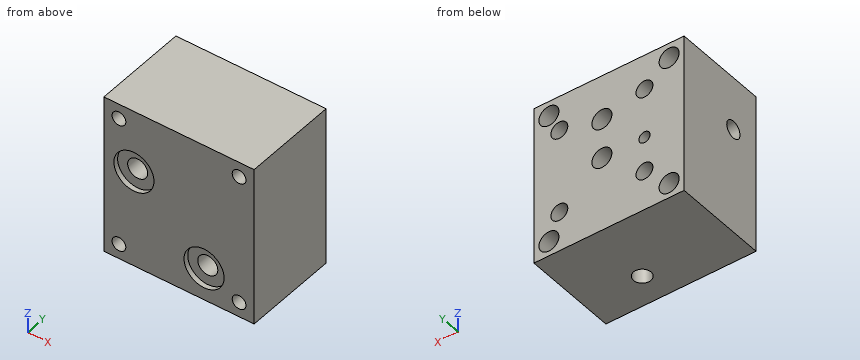
from build123d import *

# Parameters (mm, degrees)
SKETCH1_W           = 95.25
SKETCH1_H           = 101.6
BOSS_EXTRUDE1_DEPTH = 30.1625
CUT_EXTRUDE2_START  = 30.1625
SKETCH2_R           = 4.3688
CUT_EXTRUDE2_DEPTH  = 101.6
CUT_EXTRUDE4_START  = 30.1625
SKETCH3_R           = 6.35
CUT_EXTRUDE4_DEPTH  = 25.4
CUT_EXTRUDE6_START  = 30.1625
SKETCH4_R           = 5.3578125
CUT_EXTRUDE6_DEPTH  = 20.32
CUT_EXTRUDE8_START  = 30.1625
SKETCH5_R           = 6.35
CUT_EXTRUDE8_DEPTH  = 45.72
CUT_EXTRUDE10_START = 30.1625
SKETCH6_R           = 3.556
CUT_EXTRUDE10_DEPTH = 7.9375
CUT_EXTRUDE12_START = -47.625
SKETCH7_R           = 5.55625
CUT_EXTRUDE12_DEPTH = 53.34
CUT_EXTRUDE14_START = -50.8
SKETCH8_R           = 5.55625
CUT_EXTRUDE14_DEPTH = 53.34
CUT_EXTRUDE16_START = -30.1625
SKETCH9_R           = 6.35
CUT_EXTRUDE16_DEPTH = 27.94
CUT_EXTRUDE18_START = -30.1625
SKETCH10_R          = 12.7127
CUT_EXTRUDE18_DEPTH = 3.1242


with BuildPart() as part:
    # Sketch1 → Boss-Extrude1 (new, symmetric)
    with BuildSketch(Plane(origin=(0, 0, 0), x_dir=(1, 0, 0), z_dir=(0, 1, 0))):
        Rectangle(SKETCH1_W, SKETCH1_H)
    extrude(amount=BOSS_EXTRUDE1_DEPTH, both=True)

    # Sketch2 → Cut-Extrude2 (cut)
    with BuildSketch(Plane(origin=(0, 0, 0), x_dir=(1, 0, 0), z_dir=(0, 1, 0)).offset(CUT_EXTRUDE2_START)):
        with Locations(Location((-38.1, -41.275, 0), (0, 0, 270))):
            Circle(SKETCH2_R)
        with Locations(Location((38.1, -41.275, 0), (0, 0, 270))):
            Circle(SKETCH2_R)
        with Locations(Location((-38.1, 41.275, 0), (0, 0, 270))):
            Circle(SKETCH2_R)
        with Locations(Location((38.1, 41.275, 0), (0, 0, 270))):
            Circle(SKETCH2_R)
    extrude(amount=-CUT_EXTRUDE2_DEPTH, mode=Mode.SUBTRACT)

    # Sketch3 → Cut-Extrude4 (cut)
    with BuildSketch(Plane(origin=(0, 0, 0), x_dir=(1, 0, 0), z_dir=(0, 1, 0)).offset(CUT_EXTRUDE4_START)):
        with Locations(Location((-38.1, -41.275, 0), (0, 0, 270))):
            Circle(SKETCH3_R)
        with Locations(Location((38.1, -41.275, 0), (0, 0, 270))):
            Circle(SKETCH3_R)
        with Locations(Location((-38.1, 41.275, 0), (0, 0, 270))):
            Circle(SKETCH3_R)
        with Locations(Location((38.1, 41.275, 0), (0, 0, 270))):
            Circle(SKETCH3_R)
    extrude(amount=-CUT_EXTRUDE4_DEPTH, mode=Mode.SUBTRACT)

    # Sketch4 → Cut-Extrude6 (cut)
    with BuildSketch(Plane(origin=(0, 0, 0), x_dir=(1, 0, 0), z_dir=(0, 1, 0)).offset(CUT_EXTRUDE6_START)):
        with Locations(Location((-22.479, -28.575, 0), (0, 0, 270))):
            Circle(SKETCH4_R)
        with Locations(Location((31.496, -28.575, 0), (0, 0, 270))):
            Circle(SKETCH4_R)
        with Locations(Location((-22.479, 25.4, 0), (0, 0, 270))):
            Circle(SKETCH4_R)
        with Locations(Location((31.496, 25.4, 0), (0, 0, 270))):
            Circle(SKETCH4_R)
    extrude(amount=-CUT_EXTRUDE6_DEPTH, mode=Mode.SUBTRACT)

    # Sketch5 → Cut-Extrude8 (cut)
    with BuildSketch(Plane(origin=(0, 0, 0), x_dir=(1, 0, 0), z_dir=(0, 1, 0)).offset(CUT_EXTRUDE8_START)):
        with Locations(Location((4.5085, -22.225, 0), (0, 0, 270))):
            Circle(SKETCH5_R)
        with Locations(Location((4.5085, 3.175, 0), (0, 0, 270))):
            Circle(SKETCH5_R)
    extrude(amount=-CUT_EXTRUDE8_DEPTH, mode=Mode.SUBTRACT)

    # Sketch6 → Cut-Extrude10 (cut)
    with BuildSketch(Plane(origin=(0, 0, 0), x_dir=(1, 0, 0), z_dir=(0, 1, 0)).offset(CUT_EXTRUDE10_START)):
        with Locations(Location((-22.479, 3.175, 0), (0, 0, 270))):
            Circle(SKETCH6_R)
    extrude(amount=-CUT_EXTRUDE10_DEPTH, mode=Mode.SUBTRACT)

    # Sketch7 → Cut-Extrude12 (cut)
    with BuildSketch(Plane(origin=(0, 0, 0), x_dir=(0, 0, -1), z_dir=(1, 0, 0)).offset(CUT_EXTRUDE12_START)):
        with Locations(Location((-16.637, -11.1125, 0), (0, 0, 233.130102354))):
            Circle(SKETCH7_R)
    extrude(amount=CUT_EXTRUDE12_DEPTH, mode=Mode.SUBTRACT)

    # Sketch8 → Cut-Extrude14 (cut)
    with BuildSketch(Plane.XY.offset(CUT_EXTRUDE14_START)):
        with Locations(Location((10.16, -11.1125, 0), (0, 0, 233.130102354))):
            Circle(SKETCH8_R)
    extrude(amount=CUT_EXTRUDE14_DEPTH, mode=Mode.SUBTRACT)

    # Sketch9 → Cut-Extrude16 (cut)
    with BuildSketch(Plane(origin=(0, 0, 0), x_dir=(1, 0, 0), z_dir=(0, 1, 0)).offset(CUT_EXTRUDE16_START)):
        with Locations(Location((-28.575, -11.1125, 0), (0, 0, 270))):
            Circle(SKETCH9_R)
        with Locations(Location((15.875, 30.1625, 0), (0, 0, 270))):
            Circle(SKETCH9_R)
    extrude(amount=CUT_EXTRUDE16_DEPTH, mode=Mode.SUBTRACT)

    # Sketch10 → Cut-Extrude18 (cut)
    with BuildSketch(Plane(origin=(0, 0, 0), x_dir=(1, 0, 0), z_dir=(0, 1, 0)).offset(CUT_EXTRUDE18_START)):
        with Locations(Location((-28.575, -11.1125, 0), (0, 0, 270))):
            Circle(SKETCH10_R)
        with Locations(Location((15.875, 30.1625, 0), (0, 0, 270))):
            Circle(SKETCH10_R)
    extrude(amount=CUT_EXTRUDE18_DEPTH, mode=Mode.SUBTRACT)


solid = part.part
Work out the finished part from the listing and answer in its coordinate system (mm). Round coordinates to 2 decimals unless told otherwise and drop trailing zeros. Write each loop counter-clockwise with the first axis right and the second up, starting at its lowest first coordinate (ties: lowest second). Pieces come first, ordered by that corner, then holes. Notation, with made-up numbers: (-32, 76.5) - (8, 76.5) arc R31 cw to (8, 105.5) - close; hole circle Ø3 at (77, 1.25). An arc over 180 degrees is marked (long way). Answer in a Markdown table with one row per item. Add a question column.
1. A cutting plane is placed at C-C, the plane y = -21. Count the separate pieces of the cut face and the enclosed holes in it, and give its area (3 significant figures).
2. Given pin 1 (11.5 mm diameter, centred on x = 4.51, z = -3.18, fed in from +Y); pin 2 (10 mm diameter, centred on x = 10.5, y = -11.5, fed in from -Z); pin 3 (14 mm diameter, centred on x = 40, z = 39, fed in from +Y); pin 4 (5.5 mm diameter, centred on x = 33, z = -23.5, fed in from +Y), each flat-ended and moving along its own axis, determine where each tip first touches the part or whether it passes through.
3. A cutting plane is placed at D-D, the plane z = -25.4. Determine the outline of the cut face in (x, y) (1 decimal).
4. Find the intervals of material crossed by line 1 along X through (y, z) = (22.25, -25.4) (3 decimals); line 2 along X through (y, z) = (2.5, 41) (3 decimals); line 3 along Z through (x, y) = (3.5, 25), in increasing order. Write a range as from..to.
5. A cutting plane is placed at A-A, the plane x = 38.1. Determine the outline of the cut face in (y, z) (1 decimal), and give its area (3 significant figures).
6. A cutting plane is placed at B-B, the plane x = -38.1. Determine the outline of the cut face in (y, z) (1 decimal).
Worked out:
| question | item | result |
|---|---|---|
| 1 | separate pieces | 1 |
| 1 | enclosed holes | 6 |
| 1 | area | 9,180 mm^2 |
| 2 | pin 1 | y = -15.56 |
| 2 | pin 2 | z = 2.54 |
| 2 | pin 3 | y = 30.16 |
| 2 | pin 4 | y = 9.84 |
| 3 | outline | (-47.6, -30.2) - (4.1, -30.2) - (4.1, -27) - (11.7, -27) - (11.7, -16.5) arc R5.6 cw (long way) to (11.7, -5.8) - (11.7, -2.2) - (20.1, -2.2) - (20.1, -27) - (27.7, -27) - (27.7, -30.2) - (47.6, -30.2) - (47.6, 30.2) - (36.9, 30.2) - (36.9, 9.8) - (26.1, 9.8) - (26.1, 30.2) - (-17.1, 30.2) - (-17.1, 9.8) - (-27.8, 9.8) - (-27.8, 30.2) - (-47.6, 30.2) - close |
| 4 | line 1 | -47.625..-27.837, -17.121..26.138, 36.854..47.625 |
| 4 | line 2 | -47.625..-42.46, -33.74..33.74, 42.46..47.625 |
| 4 | line 3 | -50.8..-9.44, 3.09..15.96, 28.49..50.8 |
| 5 | outline | (-30.2, -50.8) - (30.2, -50.8) - (30.2, -47.6) - (4.8, -47.6) - (4.8, -45.6) - (-30.2, -45.6) - close; (-30.2, -36.9) - (4.8, -36.9) - (4.8, -34.9) - (30.2, -34.9) - (30.2, 34.9) - (4.8, 34.9) - (4.8, 36.9) - (-30.2, 36.9) - close; (-30.2, 45.6) - (4.8, 45.6) - (4.8, 47.6) - (30.2, 47.6) - (30.2, 50.8) - (-30.2, 50.8) - close |
| 5 | area | 4,870 mm^2 |
| 6 | outline | (-30.2, -50.8) - (30.2, -50.8) - (30.2, -47.6) - (4.8, -47.6) - (4.8, -45.6) - (-30.2, -45.6) - close; (-30.2, -36.9) - (4.8, -36.9) - (4.8, -34.9) - (30.2, -34.9) - (30.2, 34.9) - (4.8, 34.9) - (4.8, 36.9) - (-30.2, 36.9) - (-30.2, 19.5) - (-27, 19.5) - (-27, 2.7) - (-30.2, 2.7) - close; (-30.2, 45.6) - (4.8, 45.6) - (4.8, 47.6) - (30.2, 47.6) - (30.2, 50.8) - (-30.2, 50.8) - close; hole circle Ø11.1 at (-11.1, 16.6) |
